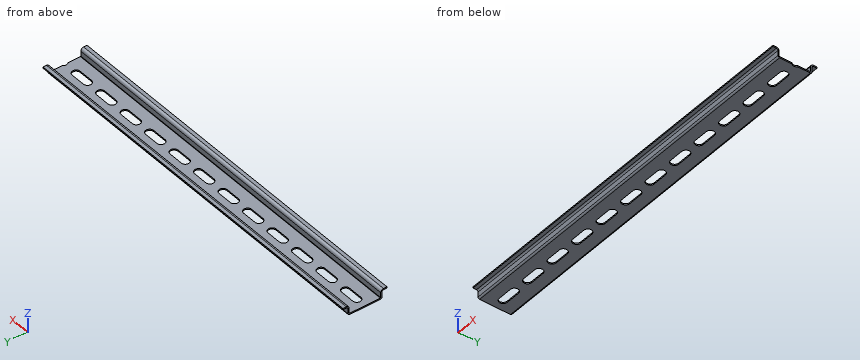
from build123d import *

# Parameters (mm, degrees)
STRUCTURAL_MEMBER1_DEPTH = 304.8
CUT_EXTRUDE1_REACH       = 155.585
LPATTERN1_COUNT          = 13
LPATTERN1_PITCH          = 24.892


with BuildPart() as part:
    # Sketch2 → Structural Member1 (new body)
    with BuildSketch(Plane(origin=(-152.4, 0, 0), x_dir=(0, 0, -1), z_dir=(1, 0, 0))):
        with BuildLine():
            Line((0, 12.25), (0, -12.25))
            ThreePointArc((0, -12.25), (-0.366116524, -13.133883476), (-1.25, -13.5))
            Line((-1.25, -13.5), (-5.25, -13.5))
            ThreePointArc((-5.25, -13.5), (-6.133883476, -13.866116524), (-6.5, -14.75))
            Line((-6.5, -14.75), (-6.5, -17.5))
            Line((-6.5, -17.5), (-7.5, -17.5))
            Line((-7.5, -17.5), (-7.5, -14.75))
            ThreePointArc((-7.5, -14.75), (-6.840990258, -13.159009742), (-5.25, -12.5))
            Line((-5.25, -12.5), (-1.25, -12.5))
            ThreePointArc((-1.25, -12.5), (-1.073223305, -12.426776695), (-1, -12.25))
            Line((-1, -12.25), (-1, 12.25))
            ThreePointArc((-1, 12.25), (-1.073223305, 12.426776695), (-1.25, 12.5))
            Line((-1.25, 12.5), (-5.25, 12.5))
            ThreePointArc((-5.25, 12.5), (-6.840990258, 13.159009742), (-7.5, 14.75))
            Line((-7.5, 14.75), (-7.5, 17.5))
            Line((-7.5, 17.5), (-6.5, 17.5))
            Line((-6.5, 17.5), (-6.5, 14.75))
            ThreePointArc((-6.5, 14.75), (-6.133883476, 13.866116524), (-5.25, 13.5))
            Line((-5.25, 13.5), (-1.25, 13.5))
            ThreePointArc((-1.25, 13.5), (-0.366116524, 13.133883476), (0, 12.25))
        make_face()
    extrude(amount=STRUCTURAL_MEMBER1_DEPTH)

    # Sketch3 → Cut-Extrude1 (cut, up to next)
    with BuildSketch(Plane.XY, mode=Mode.PRIVATE) as cut_extrude1_sk1:
        with BuildLine():
            Line((-144.145, 3.175), (-132.715, 3.175))
            ThreePointArc((-132.715, 3.175), (-129.54, 0), (-132.715, -3.175))
            Line((-132.715, -3.175), (-144.145, -3.175))
            ThreePointArc((-144.145, -3.175), (-147.32, 0), (-144.145, 3.175))
        make_face()
    cut_extrude1_tool1 = extrude(cut_extrude1_sk1.sketch, amount=CUT_EXTRUDE1_REACH, mode=Mode.PRIVATE) & part.part
    cut_extrude1 = cut_extrude1_tool1.solids().sort_by_distance((-138.43, 0, 0))[0]
    add(cut_extrude1, mode=Mode.SUBTRACT)

    # LPattern1: Cut-Extrude1 ×13
    with Locations(*[(i * LPATTERN1_PITCH, 0, 0) for i in range(1, LPATTERN1_COUNT)]):
        add(cut_extrude1, mode=Mode.SUBTRACT)


solid = part.part
For this review, take the finished solid that the model builds, in its own axes (mm). Give positions to 0.01 mm unless a question says otherwise; leave off trailing zeros. Loops run counter-clockwise (first coordinate to the right, second up) from the corner with the lowest first, then second, coordinate; pieces in that order, holes last. Notation, with made-up numbers: M 50.25,15.25 L 81.25,15.25 A30 ccw 81.25,39.25 Z; hole C -5.5,-35 d11. An arc over 180 degrees is marked long. Answer as a JSON object with one key per item and string values. Group by question number.
Q1. Insertion check: P1, Ø0.5, axis at x = 87, z = 0.5, coming from the -Y side; P2, Ø0.5, axis at x = 10, z = 0.5, coming from the +Y side; P3, Ø1.1, axis at x = 58, z = 0.5, coming from the -Y side; P4, Ø2, axis at x = -98.5, y = -14, coming from the +Z side. Each pin has a flat end and moves straight along its axis. Give the tip position at first contact, or say it passes through.
Q2. Add section A-A on x = 63. Give the boundary of the cut face in (y, z) (3 decimals).
Q3. Add section B-B on y = 9. Give the boundary of the cut face in (x, z), and give its area (3 significant figures).
Q4. For probe 1 along Y at (x, z) = (-31, 3.5); probe 2 along Z at (x, y) = (-54.5, 9); probe 3 along Y at (x, z) = (39.5, 5.75), list the stretches that pass through material, from the lowest coordinate up. Write a range as [from, to].
Checked values:
{
 "1": {"P1": "y = -13.4", "P2": "y = 13.4", "P3": "y = -13.48", "P4": "z = 7.5"},
 "2": {"outline": "M -17.5,6.5 L -14.75,6.5 A1.25 cw -13.5,5.25 L -13.5,1.25 A1.25 ccw -12.25,0 L -3.175,0 L -3.175,1 L -12.25,1 A0.25 cw -12.5,1.25 L -12.5,5.25 A2.25 ccw -14.75,7.5 L -17.5,7.5 Z; M 3.175,0 L 12.25,0 A1.25 ccw 13.5,1.25 L 13.5,5.25 A1.25 cw 14.75,6.5 L 17.5,6.5 L 17.5,7.5 L 14.75,7.5 A2.25 ccw 12.5,5.25 L 12.5,1.25 A0.25 cw 12.25,1 L 3.175,1 Z"},
 "3": {"outline": "M -152.4,0 L 152.4,0 L 152.4,1 L -152.4,1 Z", "area": "305 mm²"},
 "4": {"probe 1": "[-13.5, -12.5], [12.5, 13.5]", "probe 2": "[0, 1]", "probe 3": "[-13.6, -12.56], [12.56, 13.6]"}
}
